For this review, take the finished solid that the model builds, in its own axes (mm). A direction names the side the tool comes from. Coordinates: 2 decimals unless noted, no trailing zeros. Loops run counter-clockwise (first coordinate to the right, second up) from the corner with the lowest first, then second, coordinate; pieces in that order, holes last.
1. Take a section at A-A, the plane z = 23.5. State the section outline as (x, y) points, then the cut area to 3 significant figures.
2. Machinability: for faces 1 (the face through (65, 1.8, 14)), 2 (the face through (7.973, 1.38, -21.225)), 3 (the face through (-51, 1.8, 14)), which of the approach directions +Z, -Z, +X, -X, +Y, -Y give a long, thin tool a straight path to every point of the face, cutting with its end or side? Answer none if there is none.
3. Take a section at C-C, the plane y = 0.65. State the section outline as (x, z) points, then the cut area to 3 significant figures.
4. To check wall thickness, follow probe 1 along X at (y, z) = (2.2, 36.5); probe 2 along Z at (x, y) = (-26.5, 1.7); probe 3 along Z at (x, y) = (-40, 0.8). State the ranges of each line that lie inside material, in increasing order.
5. Clearance check with flat-ended pins moving along their axes: P1, Ø0.8, axis at x = -51, z = 27, coming from the +Y side; P2, Ø1.5, axis at x = 16.5, z = 2.5, coming from the -Y side; P3, Ø0.5, axis at y = 2.5, z = 2, coming from the -X side. State where each tip first meets the part, or that it passes through.
6. Take a section at B-B, the plane x = 4. State the section outline as (y, z) points, then the cut area to 3 significant figures.
```python
from build123d import *

# Parameters (mm, degrees)
SKETCH_1_W          = 118.3
SKETCH_1_H          = 74.6
EXTRUDE_1_DEPTH     = 2.8
SKETCH_2_W          = 2.8
SKETCH_2_H          = 74.6
CUT_EXTRUDE_1_DEPTH = 1
CUT_EXTRUDE_2_DEPTH = 130.252166362


with BuildPart() as part:
    # 草图1 → 凸台-拉伸1 (new body)
    with BuildSketch(Plane(origin=(0, 0, 0), x_dir=(1, 0, 0), z_dir=(0, 1, 0))):
        with Locations((7.144851485, -14.694158416)):
            Rectangle(SKETCH_1_W, SKETCH_1_H)
    extrude(amount=EXTRUDE_1_DEPTH)

    # 草图2 → 切除-拉伸1 (cut)
    with BuildSketch(Plane(origin=(0, 2.8, 0), x_dir=(1, 0, 0), z_dir=(0, 1, 0))):
        with Locations((64.894851485, -14.694158416)):
            Rectangle(SKETCH_2_W, SKETCH_2_H)
        with Locations((-50.605148515, -14.694158416)):
            Rectangle(SKETCH_2_W, SKETCH_2_H)
    extrude(amount=-CUT_EXTRUDE_1_DEPTH, mode=Mode.SUBTRACT)

    # 草图3 → 切除-拉伸2 (cut, through all)
    with BuildSketch(Plane(origin=(66.294851485, 0, 0), x_dir=(0, 0, -1), z_dir=(1, 0, 0))):
        Polygon((-51.994158416, 0), (-49.194158416, 2.8), (-51.994158416, 2.8), align=None)
        Polygon((22.605841584, 0), (19.805841584, 2.8), (22.605841584, 2.8), align=None)
    extrude(amount=-CUT_EXTRUDE_2_DEPTH, mode=Mode.SUBTRACT)


solid = part.part
```
Results list:
1. outline: (-52.01, 0) - (66.29, 0) - (66.29, 1.8) - (63.49, 1.8) - (63.49, 2.8) - (-49.21, 2.8) - (-49.21, 1.8) - (-52.01, 1.8) - close
1. area: 326 mm2
2. face 1: +Z, -Z, +X, +Y
2. face 2: -Z, +X, -X, +Y
2. face 3: +Z, -Z, -X, +Y
3. outline: (-52.01, -21.96) - (66.29, -21.96) - (66.29, 51.34) - (-52.01, 51.34) - close
3. area: 8,670 mm2
4. probe 1: x = -49.21 to 63.49
4. probe 2: z = -20.91 to 50.29
4. probe 3: z = -21.81 to 51.19
5. P1: stops at y = 1.8
5. P2: stops at y = 0
5. P3: stops at x = -49.21
6. outline: (0, -22.61) - (2.8, -19.81) - (2.8, 49.19) - (0, 51.99) - close
6. area: 201 mm2
